CAD build for the part. Positions are in the model's coordinates, mm. Face numbers are marked on the shaded views. A direction names the side the tool comes from. Give positions to 0.01 mm unless a question says otherwise; leave off trailing zeros. Order: outer loops, then holes, each group sorted by start corner. A loop starts at its lowest first (then second) coordinate and runs counter-clockwise, first axis right, second up.
Item 1: Which spindle directions (+Z, -Z, +X, -X, +Y, -Y) get a long thin tool onto all of the face, cutting with end or side? Do the marked faces 4 and 5. Say none if no direction does.
Item 2: Band-saw the part on A-A on z = -10.16. Give the cut face in (x, y), plus the area to 3 significant figures.
Item 3: Band-saw the part on C-C on x = 13. Give the cut face in (y, z).
Item 4: Flat gauge pins, fed straight in: P1, Ø1, axis at y = 34.5, z = -3, coming from the +X side; P2, Ø4, axis at y = 34.1, z = -2.98, coming from the +X side; P3, Ø3, axis at x = 12.5, z = -11, coming from the +Y side; P4, Ø4.5, axis at x = 13.335, z = -10.16, coming from the -Y side. Where does each tip first touch, or does it go through?
Item 5: Two-plate mould, pull along X, no slides. Class the marked faces 1, 2 and 3: released by +X, released by -X, zero draft, split by the parting line, or undercut.
Item 6: Band-saw the part on B-B on y = 26. Give the cut face in (x, z) (3 decimals).
Item 7: Wall check: L1, parallel to X at y = 18.5, z = -10.16; L2, parallel to Z at x = 13.5, y = 19.5; L3, parallel to X at y = 13, z = -8.5. Give the ranges that are in metal, low to high.
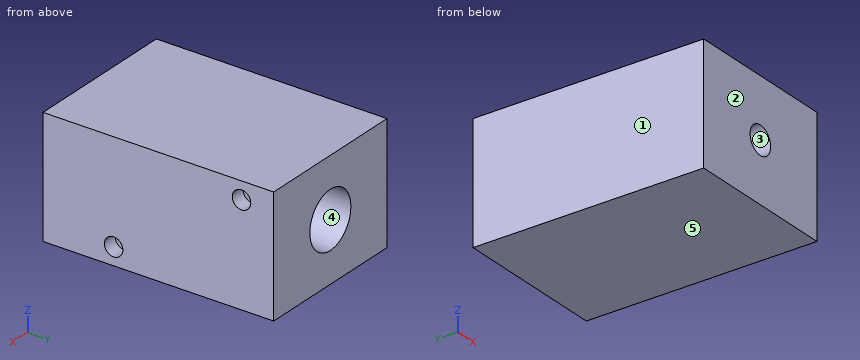
```python
from build123d import *

# Parameters (mm, degrees)
SKETCH1_W           = 26.67
SKETCH1_H           = 20.32
BOSS_EXTRUDE1_DEPTH = 39.624
SKETCH2_R           = 2.413
CUT_EXTRUDE1_DEPTH  = 40.624
SKETCH3_R           = 4.826
CUT_EXTRUDE2_DEPTH  = 28.448
SKETCH4_R           = 1.5875
CUT_EXTRUDE3_DEPTH  = 2.54


with BuildPart() as part:
    # Sketch1 → Boss-Extrude1 (new body)
    with BuildSketch(Plane(origin=(0, 0, 0), x_dir=(1, 0, 0), z_dir=(0, 1, 0))):
        with Locations((13.335, 10.16)):
            Rectangle(SKETCH1_W, SKETCH1_H)
    extrude(amount=BOSS_EXTRUDE1_DEPTH)

    # Sketch2 → Cut-Extrude1 (cut, through all)
    with BuildSketch(Plane.XZ):
        with Locations((13.335, -10.16)):
            Circle(SKETCH2_R)
    extrude(amount=-CUT_EXTRUDE1_DEPTH, mode=Mode.SUBTRACT)

    # Sketch3 → Cut-Extrude2 (cut)
    with BuildSketch(Plane(origin=(0, 39.624, 0), x_dir=(1, 0, 0), z_dir=(0, 1, 0))):
        with Locations((13.335, 10.16)):
            Circle(SKETCH3_R)
    extrude(amount=-CUT_EXTRUDE2_DEPTH, mode=Mode.SUBTRACT)

    # Sketch4 → Cut-Extrude3 (cut)
    with BuildSketch(Plane(origin=(26.67, 0, 0), x_dir=(0, 0, -1), z_dir=(1, 0, 0))):
        with Locations((2.9845, 34.0995)):
            Circle(SKETCH4_R)
        with Locations((17.3355, 12.1285)):
            Circle(SKETCH4_R)
    extrude(amount=-CUT_EXTRUDE3_DEPTH, mode=Mode.SUBTRACT)


solid = part.part
```
The answers:
1. face 4: +Y
1. face 5: -Z, +X, -X, +Y, -Y
2. outline: (0, 0) - (10.92, 0) - (10.92, 11.18) - (8.51, 11.18) - (8.51, 39.62) - (0, 39.62) - close; (15.75, 0) - (26.67, 0) - (26.67, 39.62) - (18.16, 39.62) - (18.16, 11.18) - (15.75, 11.18) - close
2. area: 728 mm2
3. outline: (0, -20.32) - (39.62, -20.32) - (39.62, -14.97) - (11.18, -14.97) - (11.18, -12.55) - (0, -12.55) - close; (0, -7.77) - (11.18, -7.77) - (11.18, -5.35) - (39.62, -5.35) - (39.62, 0) - (0, 0) - close
4. P1: stops at x = 24.13
4. P2: stops at x = 26.67
4. P3: stops at y = 11.18
4. P4: passes through
5. face 1: released by -X
5. face 2: zero draft
5. face 3: undercut
6. outline: (0, -20.32) - (26.67, -20.32) - (26.67, 0) - (0, 0) - close; hole circle Ø9.652 at (13.335, -10.16)
7. L1: x = 0 to 8.51, 18.16 to 26.67
7. L2: z = -20.32 to -14.98, -5.34 to 0
7. L3: x = 0 to 8.8, 17.87 to 26.67
